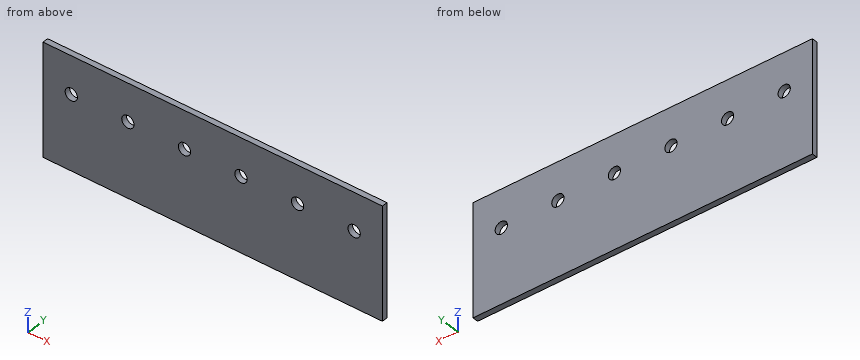
from build123d import *

# Parameters (mm, degrees)
SKIZZE1_W                       = 180
SKIZZE1_H                       = 59.5
AUFSATZ_LINEAR_AUSTRAGEN1_DEPTH = 3
SKIZZE2_R                       = 3.25
SCHNITT_LINEAR_AUSTRAGEN1_DEPTH = 3


with BuildPart() as part:
    # Skizze1 → Aufsatz-Linear austragen1 (new body)
    with BuildSketch(Plane(origin=(0, 0, 0), x_dir=(1, 0, 0), z_dir=(0, 1, 0))):
        Rectangle(SKIZZE1_W, SKIZZE1_H)
    extrude(amount=AUFSATZ_LINEAR_AUSTRAGEN1_DEPTH)

    # Skizze2 → Schnitt-Linear austragen1 (cut)
    with BuildSketch(Plane(origin=(0, 3, 0), x_dir=(1, 0, 0), z_dir=(0, 1, 0))):
        with Locations(Location((-75, -9.75, 0), (0, 0, 270))):
            Circle(SKIZZE2_R)
        with Locations(Location((-45, -9.75, 0), (0, 0, 270))):
            Circle(SKIZZE2_R)
        with Locations(Location((-15, -9.75, 0), (0, 0, 270))):
            Circle(SKIZZE2_R)
        with Locations(Location((15, -9.75, 0), (0, 0, 270))):
            Circle(SKIZZE2_R)
        with Locations(Location((45, -9.75, 0), (0, 0, 270))):
            Circle(SKIZZE2_R)
        with Locations(Location((75, -9.75, 0), (0, 0, 270))):
            Circle(SKIZZE2_R)
    extrude(amount=-SCHNITT_LINEAR_AUSTRAGEN1_DEPTH, mode=Mode.SUBTRACT)


solid = part.part
Verification items for the finished model (mm, model axes). Coordinates: 2 decimals unless noted, no trailing zeros. Order: outer loops, then holes, each group sorted by start corner. A loop starts at its lowest first (then second) coordinate and runs counter-clockwise, first axis right, second up.
Item 1: Material ranges on L1, parallel to Z at x = 16.5, y = 1.65, recorded low to high.
Filled in:
L1: z = -29.75 to 6.87, 12.63 to 29.75
Item 2: Depth check by flat-ended pin: pin 1 (5 mm diameter, centred on x = 45, z = 9.75, fed in from +Y). Enter the tip coordinate at first touch or a pass-through.
Filled in:
pin 1: passes through
Item 3: Section check C-C, the plane y = 0.65. Enter the section's corners in (x, z), then the cut area to 3 significant figures.
Filled in:
outline: (-90, -29.75) - (90, -29.75) - (90, 29.75) - (-90, 29.75) - close; hole circle Ø6.5 at (-75, 9.75); hole circle Ø6.5 at (-45, 9.75); hole circle Ø6.5 at (-15, 9.75); hole circle Ø6.5 at (15, 9.75); hole circle Ø6.5 at (45, 9.75); hole circle Ø6.5 at (75, 9.75)
area: 10,500 mm2
Item 4: Section check A-A, the plane x = -15. Enter the section's corners in (y, z).
Filled in:
outline: (0, -29.75) - (3, -29.75) - (3, 6.5) - (0, 6.5) - close; (0, 13) - (3, 13) - (3, 29.75) - (0, 29.75) - close
Item 5: Section check B-B, the plane z = 9.75. Enter the section's corners in (x, y), then the cut area to 3 significant figures.
Filled in:
outline: (-90, 0) - (-78.25, 0) - (-78.25, 3) - (-90, 3) - close; (-71.75, 0) - (-48.25, 0) - (-48.25, 3) - (-71.75, 3) - close; (-41.75, 0) - (-18.25, 0) - (-18.25, 3) - (-41.75, 3) - close; (-11.75, 0) - (11.75, 0) - (11.75, 3) - (-11.75, 3) - close; (18.25, 0) - (41.75, 0) - (41.75, 3) - (18.25, 3) - close; (48.25, 0) - (71.75, 0) - (71.75, 3) - (48.25, 3) - close; (78.25, 0) - (90, 0) - (90, 3) - (78.25, 3) - close
area: 423 mm2
